Geometry: final body of the model. Coordinates: model frame, mm. Coordinates: 2 decimals unless noted, no trailing zeros. Order: outer loops, then holes, each group sorted by start corner. A loop starts at its lowest first (then second) coordinate and runs counter-clockwise, first axis right, second up. Notation, with made-up numbers: (-21.75, -40) - (-11.75, -40) arc R21 cw to (-11.75, -3) - close; hole circle Ø1 at (-39, -38.75). An arc over 180 degrees is marked (long way). Use a Markdown table: item, result. Add a question column.
```python
from build123d import *

# Parameters (mm, degrees)
MODEL_R                 = 1.5
SALIENTE_EXTRUIR1_DEPTH = 3


with BuildPart() as part:
    # Model → Saliente-Extruir1 (new body)
    with BuildSketch(Plane.XY):
        Polygon((-105.943383637, 105.556539338), (-105.943383637, 69.556539338), (-69.943383637, 69.556539338), align=None)
        with Locations((-101.443383637, 92.056539338)):
            Circle(MODEL_R, mode=Mode.SUBTRACT)
        with Locations((-101.443383637, 83.056539338)):
            Circle(MODEL_R, mode=Mode.SUBTRACT)
        with Locations((-92.443383637, 83.056539338)):
            Circle(MODEL_R, mode=Mode.SUBTRACT)
        with Locations((-101.443383637, 74.056539338)):
            Circle(MODEL_R, mode=Mode.SUBTRACT)
        with Locations((-92.443383637, 74.056539338)):
            Circle(MODEL_R, mode=Mode.SUBTRACT)
        with Locations((-83.443383637, 74.056539338)):
            Circle(MODEL_R, mode=Mode.SUBTRACT)
    extrude(amount=SALIENTE_EXTRUIR1_DEPTH)


solid = part.part
```
1) Section query B-B (x = -83). Return the cut outline in (y, z), and give its area (3 significant figures).
2) Draft query along X for faces 1 (the cylindrical face through (-82.637, 75.321, 1.479)), 2 (the flat face through (-87.691, 87.305, 1.479)), 3 (the cylindrical face through (-91.013, 74.507, 1.479)), 4 (the flat face through (-105.943, 88, 1)). Return one class per face: released by +X, released by -X, zero draft, split by the parting line, or undercut.
3) Line query: line 1 (X direction, y = 84, z = 2.2); line 2 (X direction, y = 82, z = 2.35); line 3 (Y direction, x = -102.5, z = 2.85). Output: solid intervals per line, ascending. Write a range as from..to.
4) Section query D-D (x = -74). Return the cut outline in (y, z), and give its area (3 significant figures).
5) Section query A-A (y = 91). Return the cut outline in (x, z), and give its area (3 significant figures).
6) Section query C-C (z = 0.7). Return the cut outline in (x, y).
7) First-contact query: pin 1 (3.5 mm diameter, centred on x = -101.44, y = 92.06, fed in from +Z); pin 2 (2.5 mm diameter, centred on x = -92.44, y = 74.06, fed in from +Z). Flat tips, straight axial feed; report the tip coordinate or a pass-through.
From the geometry:
| question | item | result |
|---|---|---|
| 1 | outline | (69.56, 0) - (72.62, 0) - (72.62, 3) - (69.56, 3) - close; (75.49, 0) - (82.61, 0) - (82.61, 3) - (75.49, 3) - close |
| 1 | area | 30.6 mm^2 |
| 2 | face 1 | undercut |
| 2 | face 2 | released by +X |
| 2 | face 3 | undercut |
| 2 | face 4 | released by -X |
| 3 | line 1 | x = -105.94..-102.61, -100.28..-93.61, -91.28..-84.39 |
| 3 | line 2 | x = -105.94..-102.51, -100.38..-93.51, -91.38..-82.39 |
| 3 | line 3 | y = 69.56..72.99, 75.12..81.99, 84.12..90.99, 93.12..102.11 |
| 4 | outline | (69.56, 0) - (73.61, 0) - (73.61, 3) - (69.56, 3) - close |
| 4 | area | 12.2 mm^2 |
| 5 | outline | (-105.94, 0) - (-102.51, 0) - (-102.51, 3) - (-105.94, 3) - close; (-100.38, 0) - (-91.39, 0) - (-91.39, 3) - (-100.38, 3) - close |
| 5 | area | 37.3 mm^2 |
| 6 | outline | (-105.94, 69.56) - (-69.94, 69.56) - (-105.94, 105.56) - close; hole circle Ø3 at (-101.44, 74.06); hole circle Ø3 at (-101.44, 83.06); hole circle Ø3 at (-101.44, 92.06); hole circle Ø3 at (-92.44, 74.06); hole circle Ø3 at (-92.44, 83.06); hole circle Ø3 at (-83.44, 74.06) |
| 7 | pin 1 | stops at z = 3 |
| 7 | pin 2 | passes through |
